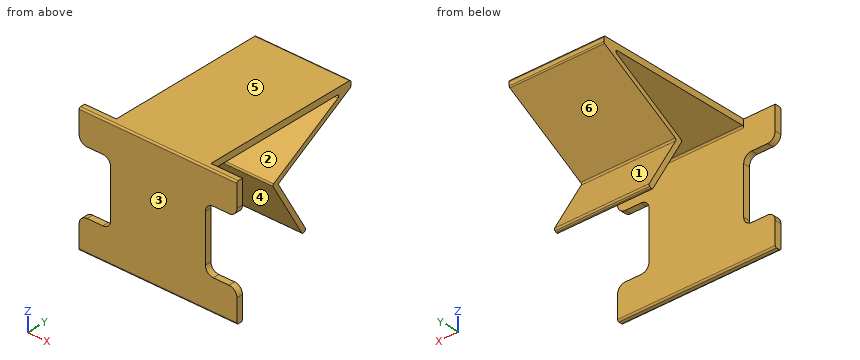
```python
from build123d import *

# Parameters (mm, degrees)
SKETCH_1_W      = 40
SKETCH_1_H      = 4
EXTRUDE_1_DEPTH = 30
EXTRUDE_2_DEPTH = 50
FILLET_1_R      = 5


with BuildPart() as part:
    # Sketch 1 → Extrude 1 (new, symmetric)
    with BuildSketch(Plane(origin=(0, 0, 0), x_dir=(0, 0, -1), z_dir=(1, 0, 0))):
        with BuildLine():
            Line((33.5, 52.904501177), (4.288675135, 103.5))
            ThreePointArc((4.288675135, 103.5), (3.922649731, 103.866025404), (3.422649731, 104))
            Line((3.422649731, 104), (1, 104))
            ThreePointArc((1, 104), (0.292893219, 103.707106781), (0, 103))
            Line((0, 103), (0, 4))
            Line((0, 4), (5, 4))
            ThreePointArc((5, 4), (4.292893219, 4.292893219), (4, 5))
            Line((4, 5), (4, 94.267949192))
            ThreePointArc((4, 94.267949192), (4.741180955, 95.233875019), (5.866025404, 94.767949192))
            Line((5.866025404, 94.767949192), (32.401923789, 48.806424965))
            ThreePointArc((32.401923789, 48.806424965), (33.009130147, 48.340499139), (33.767949192, 48.440399562))
            Line((33.767949192, 48.440399562), (69.274990748, 68.940399562))
            ThreePointArc((69.274990748, 68.940399562), (69.740916574, 69.54760592), (69.641016151, 70.306424965))
            Line((69.641016151, 70.306424965), (69.141016151, 71.172450369))
            ThreePointArc((69.141016151, 71.172450369), (68.533809793, 71.638376195), (67.774990748, 71.538475773))
            Line((67.774990748, 71.538475773), (34.866025404, 52.538475773))
            ThreePointArc((34.866025404, 52.538475773), (34.107206359, 52.43857535), (33.5, 52.904501177))
        make_face()
        with BuildLine():
            Line((5, 4), (0, 4))
            Line((0, 4), (0, 1))
            ThreePointArc((0, 1), (0.292893219, 0.292893219), (1, 0))
            Line((1, 0), (20, 0))
            Line((20, 0), (20, 4))
            Line((20, 4), (5, 4))
        make_face()
        with Locations((40, 2)):
            Rectangle(SKETCH_1_W, SKETCH_1_H)
        with BuildLine():
            Line((79, 4), (60, 4))
            Line((60, 4), (60, 0))
            Line((60, 0), (79, 0))
            ThreePointArc((79, 0), (79.707106781, 0.292893219), (80, 1))
            Line((80, 1), (80, 3))
            ThreePointArc((80, 3), (79.707106781, 3.707106781), (79, 4))
        make_face()
    extrude(amount=EXTRUDE_1_DEPTH, both=True)

    # Sketch 1_4 → Extrude 2 (add, symmetric)
    with BuildSketch(Plane(origin=(0, 0, 0), x_dir=(0, 0, -1), z_dir=(1, 0, 0))):
        with BuildLine():
            Line((5, 4), (0, 4))
            Line((0, 4), (0, 1))
            ThreePointArc((0, 1), (0.292893219, 0.292893219), (1, 0))
            Line((1, 0), (20, 0))
            Line((20, 0), (20, 4))
            Line((20, 4), (5, 4))
        make_face()
        with BuildLine():
            Line((79, 4), (60, 4))
            Line((60, 4), (60, 0))
            Line((60, 0), (79, 0))
            ThreePointArc((79, 0), (79.707106781, 0.292893219), (80, 1))
            Line((80, 1), (80, 3))
            ThreePointArc((80, 3), (79.707106781, 3.707106781), (79, 4))
        make_face()
    extrude(amount=EXTRUDE_2_DEPTH, both=True)

    # Fillet 1
    fillet_1_edges = [part.edges().sort_by_distance(p)[0] for p in [
        (30, 2, -60),
        (-30, 2, -60),
        (-50, 2, -60),
        (50, 2, -60),
        (-30, 2, -20),
        (30, 2, -20),
        (50, 2, -20),
        (-50, 2, -20),
    ]]
    fillet(fillet_1_edges, radius=FILLET_1_R)


solid = part.part
```
The listing builds one solid part. Answer for the finished solid, in the listing's coordinates (mm). Face numbers are marked on the shaded views. A direction names the side the tool comes from. Coordinates: 2 decimals unless noted, no trailing zeros. Write each loop counter-clockwise with the first axis right and the second up, starting at its lowest first coordinate (ties: lowest second). Pieces come first, ordered by that corner, then holes. Notation, with made-up numbers: (68, -10) - (92, -10) arc R21 cw to (92, 2) - close; hole circle Ø4 at (76, 27). An arc over 180 degrees is marked (long way). Return JSON: item names as keys, results as strings. Group by question number.
Q1. Flat-ended cylindrical pins translate along their axes: pin 1 Ø2 at (x, z) = (24.5, -25.5) entering from +Y; pin 2 Ø21 at (y, z) = (61, -18) entering from +X; pin 3 Ø4.5 at (y, z) = (2.5, -40) entering from -X. Find the tip coordinate at first contact, or state that the pin passes through.
Q2. For a pull along Y with two mould halves and no side action, classify the marked faces 4, 5 and 6 as +Y half, -Y half, draft (parallel to the pull), parting line (faces both ways), or undercut.
Q3. The part is cut by section A-A on x = 41. Write down the section's boundary in (y, z).
Q4. The part is cut by section B-B on y = 55. Write down the section's boundary in (x, z), and give its area (3 significant figures).
Q5. The part is cut by section D-D on y = 79. Write down the section's boundary in (x, z).
Q6. The part is cut by section C-C on z = -23. Write down the section's boundary in (x, y), and give its area (3 significant figures).
Q7. Which of the six approach directions +Z, -Z, +X, -X, +Y, -Y give full straight-line access (tool end or side, diameter ignored) to the marked faces 1, 2 and 3?
Q8. Find the intervals of material crossed by line 1 along Z through (x, y) = (13, 57); line 2 along Z through (x, y) = (-19, 59); line 3 along Y through (x, z) = (-38, -3), in increasing order. Write a range as [from, to].
Evaluation:
{
 "1": {"pin 1": "stops at y = 68.49", "pin 2": "stops at x = 30", "pin 3": "stops at x = -30"},
 "2": {"face 4": "undercut", "face 5": "draft", "face 6": "+Y half"},
 "3": {"outline": "(0, -79) arc R1 ccw to (1, -80) - (3, -80) arc R1 ccw to (4, -79) - (4, -60) - (0, -60) - close; (0, -20) - (4, -20) - (4, 0) - (1, 0) arc R1 ccw to (0, -1) - close"},
 "4": {"outline": "(-30, -45.13) - (30, -45.13) - (30, -39.13) - (-30, -39.13) - close; (-30, -32.29) - (30, -32.29) - (30, -28.83) - (-30, -28.83) - close; (-30, -4) - (30, -4) - (30, 0) - (-30, 0) - close", "area": "808 mm2"},
 "5": {"outline": "(-30, -18.43) - (30, -18.43) - (30, -14.97) - (-30, -14.97) - close; (-30, -4) - (30, -4) - (30, 0) - (-30, 0) - close"},
 "6": {"outline": "(-30.42, 0) - (30.42, 0) - (30.42, 4) - (-30.42, 4) - close; (-30, 65.09) - (30, 65.09) - (30, 71.09) - (-30, 71.09) - close", "area": "603 mm2"},
 "7": {"face 1": "+X, -X, +Y", "face 2": "+X, -X", "face 3": "+Z, -Z, +X, -X, -Y"},
 "8": {"line 1": "z = [-48.59, -42.59], [-31.14, -27.67], [-4, 0]", "line 2": "z = [-52.06, -46.06], [-29.98, -26.52], [-4, 0]", "line 3": "y = [0, 4]"}
}
